Could you check a few things on this model? Use its own coordinates, in mm. A direction names the side the tool comes from. Round coordinates to 2 decimals unless told otherwise and drop trailing zeros. Write each loop counter-clockwise with the first axis right and the second up, starting at its lowest first coordinate (ties: lowest second). Pieces come first, ordered by that corner, then holes. Notation, with made-up numbers: (66.5, 29.5) -> (108.5, 29.5) arc R16 ccw to (108.5, 60.5) -> close; hole circle Ø7 at (50, 32). An arc over 180 degrees is marked (long way). One line per question, with ' | ' between items. Start each with the question number.
1. Imagine slicing it at A-A, the plane z = -5. List the corners of the cut face in (x, y) for me, and give its area (3 significant figures).
2. Imagine slicing it at D-D, the plane z = 13. List the corners of the cut face in (x, y) for me.
3. Imagine slicing it at B-B, the plane y = -63.5. List the corners of the cut face in (x, z) for me.
4. Thinking about a two-plate mould opening in Y: for faces 4 (the cylindrical face through (44.672, -74.751, -31.036)), 5 (the flat face through (8, -64.834, -13)), 6 (the flat face through (8, -66.04, 22)), 7 (the flat face through (-30.001, -30, 1)), which applies, released by +Y, released by -Y, zero draft, split by the parting line, or undercut?
5. Imagine slicing it at C-C, the plane x = 12.5. List the corners of the cut face in (y, z) for me.
6. If I drill on line 1 along Z through (x, y) = (-15.5, -64); line 2 along Z through (x, y) = (2, -63); line 3 along X through (y, z) = (-13, 12), over which ranges is the centre line in solid material (lowest first)? Write a range as [from, to].
7. For faces 1 (the cylindrical face through (44.672, -74.751, 28.731)), 2 (the flat face through (-29.13, -68.85, -6.27)), 3 (the flat face through (8, -56, 25.423)), which set-ups out of +Z, -Z, +X, -X, +Y, -Y let a thin tool reach every point of the face, with its end or its side?
from build123d import *

# Parameters (mm, degrees)
F0_W     = 76.2
F0_H     = 76.2
F1_DEPTH = 45.72
F2_W     = 76.2
F2_H     = 12.7
F3_DEPTH = 30.48
F4_W     = 76.2
F4_H     = 10.16
F5_DEPTH = 6.35
F7_DEPTH = 30.48
F8_W     = 77.3755078257
F8_H     = 11.3661354303
F9_DEPTH = 10.16
F10_R    = 5.08
F12_D    = 25.4


with BuildPart() as f1:
    # F0 (on Front) → F1 (new body)
    with BuildSketch(Plane.XZ):
        with Locations((8.099174127, 0.0226207582)):
            Rectangle(F0_W, F0_H)
    extrude(amount=F1_DEPTH)

    # F2 (on face) → F3 (join)
    with BuildSketch(Plane.XZ.offset(45.72)):
        with Locations((8.099174127, 31.7726207582)):
            Rectangle(F2_W, F2_H)
    extrude(amount=F3_DEPTH)

    # F4 (on face) → F5 (join)
    with BuildSketch(Plane(origin=(0, 0, 25.4226207582), x_dir=(1, 0, 0), z_dir=(0, 0, -1))):
        with Locations((8.099174127, 71.12)):
            Rectangle(F4_W, F4_H)
    extrude(amount=F5_DEPTH)

    # F6 (on face) → F7 (join)
    with BuildSketch(Plane.XZ.offset(45.72)):
        Polygon((-30.000825873, -11.1981863156), (-30.000825873, -38.0773792418), (46.199174127, -38.0773792418), (46.199174127, -24.6343022456), align=None)
    extrude(amount=F7_DEPTH)

    # F8 (on face) → F9 (join)
    with BuildSketch(Plane(origin=(-2.8196382357, 0, -15.9909630638), x_dir=(0.984807753, 0, -0.1736481777), z_dir=(0.1736481777, 0, 0.984807753))):
        with Locations((11.0872526432, -70.5169322848)):
            Rectangle(F8_W, F8_H)
    extrude(amount=F9_DEPTH)

    # F10
    f10_edges = [f1.edges().sort_by_distance(p)[0] for p in [
        (-30.000826, -76.2, 28.597621),
        (-30.000826, -76.2, -24.637783),
        (46.199174, -76.2, -31.355841),
        (47.081307, -76.2, -19.631479),
        (46.199174, -76.2, 28.597621),
        (46.199174, 0, 0.022621),
        (-30.000826, 0, 0.022621),
    ]]
    fillet(f10_edges, radius=F10_R)

    # F12 (through all)
    with Locations(Plane.XY.offset(38.1226207582)):
        with Locations((8.099174127, -21.8078975493)):
            Hole(F12_D / 2)


solid = f1.part
Geometry results:
1) outline: (-30, -45.72) -> (46.2, -45.72) -> (46.2, -5.08) arc R5.08 ccw to (41.12, 0) -> (-24.92, 0) arc R5.08 ccw to (-30, -5.08) -> close; (-28.91, -74.27) arc R5.08 ccw to (-24.92, -76.2) -> (-6.64, -76.2) -> (-6.64, -64.83) -> (-28.91, -64.83) -> close; hole circle Ø25.4 at (8.1, -21.81) | area: 3,220 mm2
2) outline: (-30, -45.72) -> (46.2, -45.72) -> (46.2, -5.08) arc R5.08 ccw to (41.12, 0) -> (-24.92, 0) arc R5.08 ccw to (-30, -5.08) -> close; hole circle Ø25.4 at (8.1, -21.81)
3) outline: (-30, -38.08) -> (46.2, -38.08) -> (46.2, -24.63) -> (-30, -11.2) -> close; (-30, 25.42) -> (46.2, 25.42) -> (46.2, 38.12) -> (-30, 38.12) -> close
4) face 4: released by -Y | face 5: undercut | face 6: undercut | face 7: zero draft
5) outline: (-76.2, -38.08) -> (-33.72, -38.08) -> (-33.72, 38.12) -> (-76.2, 38.12) -> (-76.2, 19.07) -> (-66.04, 19.07) -> (-66.04, 25.42) -> (-45.72, 25.42) -> (-45.72, -18.69) -> (-64.83, -18.69) -> (-64.83, -8.38) -> (-76.2, -8.38) -> close; (-9.89, -38.08) -> (0, -38.08) -> (0, 38.12) -> (-9.89, 38.12) -> close
6) line 1: z = [-38.08, -13.76], [25.42, 38.12] | line 2: z = [-38.08, -16.84], [25.42, 38.12] | line 3: x = [-30, -1.05], [17.25, 46.2]
7) face 1: +Z, +X, -Y | face 2: -X, -Y | face 3: +X, -X
